Source: CAD feature listing. Evaluate the final solid. Frame: model axes, mm. A direction names the side the tool comes from. Round coordinates to 2 decimals unless told otherwise and drop trailing zeros. Loops run counter-clockwise (first coordinate to the right, second up) from the corner with the lowest first, then second, coordinate; pieces in that order, holes last.
Item 1: Pull-direction query (X, two-part tool) for faces 5 (the cylindrical face through (-18.21, 10.897, -5.211)), 6 (the flat face through (10.1, 4.5, 7.7)), 7 (the cylindrical face through (24, 0, 15)); classes: released by +X, released by -X, zero draft, split by the parting line, or undercut.
Item 2: Section query D-D on z = 39. Return loops of the section in (x, y).
Item 3: Ray query, L1, parallel to Y at x = 17, z = -2.9; L2, parallel to Y at x = -21.5, z = 32.75; L3, parallel to X at y = 0.5, z = 25. Return the intervals inside material, ascending.
Item 4: Section query A-A on x = 0. Return loops of the section in (y, z), then the cut area to 3 significant figures.
Item 5: Section query B-B on z = 15.5. Return loops of the section in (x, y), then the cut area to 3 significant figures.
Item 6: Access query for faces 1 (the flat face through (-15, -11, -4.4)), 2 (the flat face through (-20, 1, 22)), 3 (the cylindrical face through (-24, 0, 27)), 4 (the flat face through (10.1, -4.5, 7.7)). Directions: +Z, -Z, +X, -X, +Y, -Y. A direction counts if a zero-diameter tool reaches every point of the face in a straight line with its end or side. Return the directions, or none.
Item 7: First-contact query: P1, Ø6, axis at x = 27, y = 13, coming from the +Z side; P2, Ø3, axis at x = -22, y = 0.5, coming from the +Z side; P3, Ø23.5, axis at x = 2, z = 33, coming from the +Y side; P4, Ø8, axis at x = -7, y = 3, coming from the +Z side. Flat tips, straight axial feed; report the tip coordinate or a pass-through.
Item 8: Section query C-C on y = 9. Return loops of the section in (x, z), then the cut area to 3 significant figures.
```python
from build123d import *

# Parameters (mm, degrees)
SKETCH1_R                                          = 24
BOSS_EXTRUDE1_DEPTH                                = 6
BOSS_EXTRUDE2_DEPTH                                = 4.5
BOSS_EXTRUDE2_DEPTH_BACK                           = 4.5
CHAMBRAGE_POUR_VIS_T_TE_HEXAGONALE_M42_D           = 4.5
CHAMBRAGE_POUR_VIS_T_TE_HEXAGONALE_M42_CBORE_D     = 8
CHAMBRAGE_POUR_VIS_T_TE_HEXAGONALE_M42_CBORE_DEPTH = 4.4
CHAMBRAGE_POUR_VIS_T_TE_HEXAGONALE_M31_D           = 3.4
CHAMBRAGE_POUR_VIS_T_TE_HEXAGONALE_M31_DEPTH       = 21
CHAMBRAGE_POUR_VIS_T_TE_HEXAGONALE_M31_CBORE_D     = 6.5
CHAMBRAGE_POUR_VIS_T_TE_HEXAGONALE_M31_CBORE_DEPTH = 15.4
TROU_POUR_TARAUDAGE_POUR_TROU_TARAUD_M3_D          = 2.5
TROU_POUR_TARAUDAGE_POUR_TROU_TARAUD_M3_DEPTH      = 10
TROU_POUR_TARAUDAGE_POUR_TROU_TARAUD_M3_TIP        = 0.751075774
ESQUISSE8_OUTSIDE_W                                = 69.572
ESQUISSE8_OUTSIDE_H                                = 67.572
ESQUISSE8_OUTSIDE_R                                = 24
ENL_V_MAT_EXTRU_3_DEPTH                            = 49.0000001
ENL_V_MAT_EXTRU_3_DEPTH_BACK                       = 7
BOSS_EXTRU_1_DEPTH                                 = 6
TROU_POUR_TARAUDAGE_POUR_TROU_TARAUD_M6_D          = 5


with BuildPart() as part:
    # Sketch1 → Boss-Extrude1 (new body)
    with BuildSketch(Plane.XY):
        Circle(SKETCH1_R)
    extrude(amount=-BOSS_EXTRUDE1_DEPTH)

    # Sketch2 → Boss-Extrude2 (add, two sides)
    with BuildSketch(Plane(origin=(0, 0, 0), x_dir=(1, 0, 0), z_dir=(0, 1, 0))) as boss_extrude2_sk:
        with BuildLine():
            Line((-18.02227788, -24), (-24.979991994, -24))
            ThreePointArc((-24.979991994, -24), (0.50010007, -47.994997498), (25, -23))
            Line((25, -23), (25, 6))
            Line((25, 6), (-25, 6))
            Line((-25, 6), (-25, -22))
            Line((-25, -22), (-18.02227788, -22))
            ThreePointArc((-18.02227788, -22), (0.500192092, -4.956931861), (18.05, -23))
            ThreePointArc((18.05, -23), (0.500192092, -41.043068139), (-18.02227788, -24))
        make_face()
    extrude(amount=BOSS_EXTRUDE2_DEPTH)
    extrude(boss_extrude2_sk.sketch, amount=-BOSS_EXTRUDE2_DEPTH_BACK)

    # Chambrage pour vis à tête hexagonale M42 (through all)
    with Locations(Plane.XY):
        with Locations((17, 9), (-17, -9), (-17, 9), (17, -9)):
            CounterBoreHole(CHAMBRAGE_POUR_VIS_T_TE_HEXAGONALE_M42_D / 2, CHAMBRAGE_POUR_VIS_T_TE_HEXAGONALE_M42_CBORE_D / 2, CHAMBRAGE_POUR_VIS_T_TE_HEXAGONALE_M42_CBORE_DEPTH)

    # Chambrage pour vis à tête hexagonale M31
    with Locations(Plane(origin=(0, 0, 44), x_dir=(-1, 0, 0), z_dir=(0, 0, 1))):
        with Locations((21.5, 0)):
            CounterBoreHole(CHAMBRAGE_POUR_VIS_T_TE_HEXAGONALE_M31_D / 2, CHAMBRAGE_POUR_VIS_T_TE_HEXAGONALE_M31_CBORE_D / 2, CHAMBRAGE_POUR_VIS_T_TE_HEXAGONALE_M31_CBORE_DEPTH, depth=CHAMBRAGE_POUR_VIS_T_TE_HEXAGONALE_M31_DEPTH)

    # Trou pour taraudage pour trou taraudé M31
    with Locations(Plane.XY.offset(22)):
        with Locations((-21.5, 0)):
            Hole(TROU_POUR_TARAUDAGE_POUR_TROU_TARAUD_M3_D / 2, depth=TROU_POUR_TARAUDAGE_POUR_TROU_TARAUD_M3_DEPTH)
            with Locations((0, 0, -(TROU_POUR_TARAUDAGE_POUR_TROU_TARAUD_M3_DEPTH + TROU_POUR_TARAUDAGE_POUR_TROU_TARAUD_M3_TIP / 2))):  # 118° drill point
                Cone(0, TROU_POUR_TARAUDAGE_POUR_TROU_TARAUD_M3_D / 2, TROU_POUR_TARAUDAGE_POUR_TROU_TARAUD_M3_TIP, mode=Mode.SUBTRACT)

    # Esquisse8 outside → Enlèv. mat.-Extru.3 (cut, two sides)
    with BuildSketch(Plane.XY) as enl_v_mat_extru_3_sk:
        Rectangle(ESQUISSE8_OUTSIDE_W, ESQUISSE8_OUTSIDE_H)
        Circle(ESQUISSE8_OUTSIDE_R, mode=Mode.SUBTRACT)
    extrude(amount=ENL_V_MAT_EXTRU_3_DEPTH, mode=Mode.SUBTRACT)
    extrude(enl_v_mat_extru_3_sk.sketch, amount=-ENL_V_MAT_EXTRU_3_DEPTH_BACK, mode=Mode.SUBTRACT)

    # Esquisse9 → Boss.-Extru.1 (add)
    with BuildSketch(Plane(origin=(0, 0, -6), x_dir=(-1, 0, 0), z_dir=(0, 0, -1))):
        with BuildLine():
            ThreePointArc((-28.675, 4.82124206), (-35, 0), (-28.675, -4.82124206))
            ThreePointArc((-28.675, -4.82124206), (-25.033036693, -5.211718832), (-22.634482759, -7.979986858))
            ThreePointArc((-22.634482759, -7.979986858), (-24, 0), (-22.634482759, 7.979986858))
            ThreePointArc((-22.634482759, 7.979986858), (-25.033036693, 5.211718832), (-28.675, 4.82124206))
        make_face()
    extrude(amount=-BOSS_EXTRU_1_DEPTH)

    # Trou pour taraudage pour trou taraudé M62 (through all)
    with Locations(Plane.XY):
        with Locations((30, 0)):
            Hole(TROU_POUR_TARAUDAGE_POUR_TROU_TARAUD_M6_D / 2)


solid = part.part
```
Data:
1. face 5: undercut
1. face 6: zero draft
1. face 7: released by +X
2. outline: (-19.21, -4.5) - (-8.35, -4.5) - (-8.35, 4.5) - (-19.21, 4.5) - (-19.21, 2.31) arc R3.25 cw to (-19.21, -2.31) - close; (8.35, -4.5) - (19.21, -4.5) - (19.21, 4.5) - (8.35, 4.5) - close
3. L1: y = -16.94 to -13, -5 to 5, 13 to 16.94
3. L2: y = -4.5 to -3.25, 3.25 to 4.5
3. L3: x = -23.99 to -23.12, -19.88 to -17.94, 17.94 to 23.99
4. outline: (-24, -6) - (24, -6) - (24, 0) - (4.5, 0) - (4.5, 4.95) - (-4.5, 4.95) - (-4.5, 0) - (-24, 0) - close; (-4.5, 41.05) - (4.5, 41.05) - (4.5, 48) - (-4.5, 48) - close
4. area: 395 mm2
5. outline: (-23.57, -4.5) - (-16.42, -4.5) - (-16.42, 4.5) - (-23.57, 4.5) arc R24 ccw to start; (16.42, -4.5) - (23.57, -4.5) arc R24 ccw to (23.57, 4.5) - (16.42, 4.5) - close; hole circle Ø2.5 at (-21.5, 0)
5. area: 129 mm2
6. face 1: +Z
6. face 2: -X, +Y, -Y
6. face 3: +Z, -Z, -X
6. face 4: +Z, +X, -X, -Y
7. P1: passes through
7. P2: stops at z = 28.6
7. P3: stops at y = 4.5
7. P4: stops at z = 47.82
8. outline: (-22.25, -6) - (-19.25, -6) - (-19.25, -4.4) - (-21, -4.4) - (-21, 0) - (-22.25, 0) - close; (-14.75, -6) - (14.75, -6) - (14.75, -4.4) - (13, -4.4) - (13, 0) - (-13, 0) - (-13, -4.4) - (-14.75, -4.4) - close; (19.25, -6) - (22.25, -6) - (22.25, 0) - (21, 0) - (21, -4.4) - (19.25, -4.4) - close
8. area: 182 mm2
